Input: part model. Units: mm. Frame: model coordinates. Face numbers are marked on the shaded views. Round coordinates to 2 decimals unless told otherwise and drop trailing zeros. Loops run counter-clockwise (first coordinate to the right, second up) from the corner with the lowest first, then second, coordinate; pieces in that order, holes last. Notation, with made-up numbers: (25, 61.5) - (80, 61.5) arc R11 cw to (80, 81.5) - close; hole circle Ø2 at (41.5, 42). An arc over 180 degrees is marked (long way). Write each question's results on one line, items separated by ' | '.
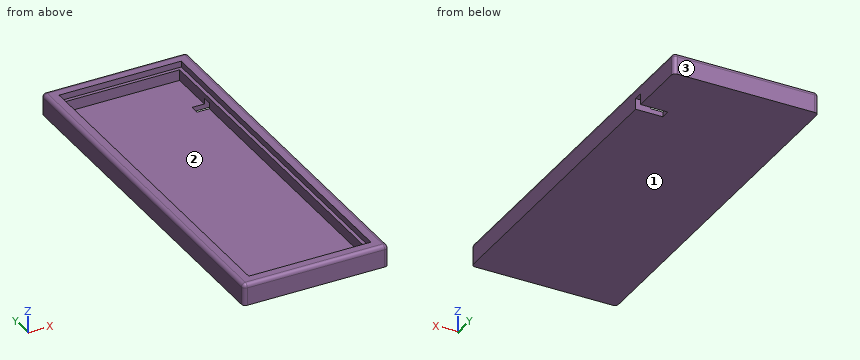
Autodesk Inventor part; units mm, degrees
ref_plane "YZ Plane" through (0, 0, 0) normal (1, 0, 0) x (0, 1, 0)
ref_plane "XZ Plane" through (0, 0, 0) normal (0, 1, 0) x (-1, 0, 0)
ref_plane "XY Plane" through (0, 0, 0) normal (0, 0, 1) x (1, 0, 0)
ref_plane "Work Plane1" through (0, 0, 0) normal (0, 0, 1) x (1, 0, 0)
sketch "Sketch3" plane through (0, 0, 0) normal (0, 0, 1) x (1, 0, 0)
  line L0 (-60.325, -155.575) -> (60.325, -155.575)
  line L1 (60.325, -155.575) -> (60.325, 155.575)
  line L2 (60.325, 155.575) -> (-60.325, 155.575)
  line L3 (-60.325, 155.575) -> (-60.325, -155.575)
  line L4 (-60.325, -155.575) -> (60.325, 155.575) construction
  line L5 (60.325, -155.575) -> (-60.325, 155.575) construction
  point P0 (0, 0)
  dimension "d4" = 120.65
  dimension "d5" = 311.15
extrude "Extrusion2" add sketch "Sketch3" against normal blind 18
sketch "Sketch4" plane through (0, 0, 0) normal (0, 0, 1) x (1, 0, 0)
  line L0 (-50.8, -146.05) -> (50.8, -146.05)
  line L1 (50.8, -146.05) -> (50.8, 146.05)
  line L2 (50.8, 146.05) -> (-50.8, 146.05)
  line L3 (-50.8, 146.05) -> (-50.8, -146.05)
  line L4 (-50.8, -146.05) -> (50.8, 146.05) construction
  line L5 (50.8, -146.05) -> (-50.8, 146.05) construction
  point P0 (0, 0)
  dimension "d8" = 101.6
  dimension "d9" = 292.1
extrude "Extrusion3" cut sketch "Sketch4" against normal blind 5
sketch "Sketch5" plane through (0, 0, -5) normal (0, 0, 1) x (1, 0, 0)
  line L0 (50.8, 146.05) -> (50.8, -146.05)
  line L1 (-50.8, 146.05) -> (50.8, 146.05)
  line L2 (-50.8, -146.05) -> (-50.8, 146.05)
  line L3 (50.8, -146.05) -> (-50.8, -146.05)
  line L4 (47.8, -143.05) -> (47.8, 143.05)
  line L5 (47.8, 143.05) -> (-47.8, 143.05)
  line L6 (-47.8, 143.05) -> (-47.8, -143.05)
  line L7 (-47.8, -143.05) -> (47.8, -143.05)
  point P0 (0, 0)
  dimension "d12" = 3
extrude "Extrusion4" cut sketch "Sketch5" against normal blind 9 contours L7 L6 L5 L4
sketch "Sketch6" plane through (0, 0, -14) normal (0, 0, 1) x (1, 0, 0)
  line L0 (47.8, 143.05) -> (47.8, -143.05)
  line L1 (47.8, 143.05) -> (47.8, -143.05)
  line L2 (47.8, 104.95) -> (37.64, 104.95)
  line L3 (37.64, 104.95) -> (37.64, 97.33)
  line L4 (37.64, 97.33) -> (47.8, 97.33)
  line L5 (47.8, 97.33) -> (47.8, 104.95)
  line L6 (-47.8, 143.05) -> (47.8, 143.05)
  line L7 (47.8, 97.33) -> (60.325, 97.33)
  line L8 (60.325, 155.575) -> (60.325, -155.575)
  line L9 (60.325, 104.95) -> (47.8, 104.95)
  point P0 (0, 0)
  dimension "d16" = 10.16
  dimension "d17" = 7.62
  dimension "d18" = 38.1
extrude "Extrusion5" cut sketch "Sketch6" along normal mid plane 10.16
fillet "Fillet1" radius 3.175 8 edges at (0, 155.575, 0) (60.325, 0, 0) (0, -155.575, 0) (-60.325, 0, 0) (-60.325, 155.575, -9) (-60.325, -155.575, -9) (60.325, -155.575, -9) (60.325, 155.575, -9)
properties part number "Case Parts"
1. Line query: line 1 (Y direction, x = 45, z = -6) (3 decimals); line 2 (X direction, y = 22, z = -7.5) (3 decimals); line 3 (X direction, y = 139, z = -4.75) (3 decimals). Output: solid intervals per line, ascending. Write a range as [from, to].
Answer:
line 1: [-155.575, -143.05], [143.05, 155.575] | line 2: [-60.325, -47.8], [47.8, 60.325] | line 3: [-60.325, -50.8], [50.8, 60.325]
2. Contact query for flat-ended pins moving along their axis: pin 1 (1.5 mm diameter, centred on x = -16, z = -2, fed in from -Y); pin 2 (2.5 mm diameter, centred on x = 54, y = 102.5, fed in from -Z); pin 3 (1.2 mm diameter, centred on y = 101.5, z = -16.5, fed in from +X). Output: stop coordinate, or through.
Answer:
pin 1: y = -155.55 | pin 2: z = -8.92 | pin 3: x = 37.64
3. Section query B-B, the plane y = 123. Output: boundary loops of the cut face in (x, z) (3 decimals), plus the area to 3 significant figures.
Answer:
outline: (-60.325, -18) - (60.325, -18) - (60.325, -3.175) arc R3.175 ccw to (57.15, 0) - (50.8, 0) - (50.8, -5) - (47.8, -5) - (47.8, -14) - (-47.8, -14) - (-47.8, -5) - (-50.8, -5) - (-50.8, 0) - (-57.15, 0) arc R3.175 ccw to (-60.325, -3.175) - close | area: 799 mm^2
4. Section query A-A, the plane x = 1. Output: boundary loops of the cut face in (y, z) (3 decimals), plus the area to 3 significant figures.
Answer:
outline: (-155.575, -18) - (155.575, -18) - (155.575, -3.175) arc R3.175 ccw to (152.4, 0) - (146.05, 0) - (146.05, -5) - (143.05, -5) - (143.05, -14) - (-143.05, -14) - (-143.05, -5) - (-146.05, -5) - (-146.05, 0) - (-152.4, 0) arc R3.175 ccw to (-155.575, -3.175) - close | area: 1,560 mm^2
5. Mould query, pull axis Y, two halves, no side actions, for the marked faces 1, 2 and 3. Classes: pulls with the +Y half, pulls with the -Y half, needs draft (parallel to the pull), parting line crosses it, or undercut.
Answer:
face 1: needs draft | face 2: undercut | face 3: pulls with the +Y half
